```python
from build123d import *

# Parameters (mm, degrees)
CYLINDER011_R     = 1.375
CYLINDER011_DEPTH = 1.4
CYLINDER012_R     = 1.375
CYLINDER012_DEPTH = 1.4
CYLINDER013_R     = 1.375
CYLINDER013_DEPTH = 1.4
CYLINDER010_R     = 1.375
CYLINDER010_DEPTH = 1.4
BOX006_W          = 56
BOX006_H          = 85
BOX006_DEPTH      = 1.4
FILLET002_R       = 3


with BuildPart() as cylinder011:
    # Cylinder011 → Cylinder011 (new body)
    with BuildSketch(Plane(origin=(52.5, 81.5, 9), x_dir=(1, 0, 0), z_dir=(0, 0, 1))):
        Circle(CYLINDER011_R)
    extrude(amount=CYLINDER011_DEPTH)


with BuildPart() as cylinder012:
    # Cylinder012 → Cylinder012 (new body)
    with BuildSketch(Plane(origin=(52.5, 23.5, 9), x_dir=(1, 0, 0), z_dir=(0, 0, 1))):
        Circle(CYLINDER012_R)
    extrude(amount=CYLINDER012_DEPTH)


with BuildPart() as cylinder013:
    # Cylinder013 → Cylinder013 (new body)
    with BuildSketch(Plane(origin=(3.5, 23.5, 9), x_dir=(1, 0, 0), z_dir=(0, 0, 1))):
        Circle(CYLINDER013_R)
    extrude(amount=CYLINDER013_DEPTH)


with BuildPart() as pi_board_holes:
    # Cylinder010 → Cylinder010 (new body)
    with BuildSketch(Plane(origin=(3.5, 81.5, 9), x_dir=(1, 0, 0), z_dir=(0, 0, 1))):
        Circle(CYLINDER010_R)
    extrude(amount=CYLINDER010_DEPTH)

    # Fusion003: union Cylinder011, Cylinder012, Cylinder013
    add(cylinder011.part)
    add(cylinder012.part)
    add(cylinder013.part)


with BuildPart() as pi_base_board:
    # Box006 → Box006 (new body)
    with BuildSketch(Plane.XY.offset(9)):
        with Locations((28, 42.5)):
            Rectangle(BOX006_W, BOX006_H)
    extrude(amount=BOX006_DEPTH)

    # Fillet002
    fillet002_edges = [pi_base_board.edges().sort_by_distance(p)[0] for p in [
        (0, 0, 9.7),
        (0, 85, 9.7),
        (56, 0, 9.7),
        (56, 85, 9.7),
    ]]
    fillet(fillet002_edges, radius=FILLET002_R)

    # Cut002: cut Pi Board Holes
    add(pi_board_holes.part, mode=Mode.SUBTRACT)


with BuildPart() as pi_base_board_1:
    # Cut002 placement: moved
    add(pi_base_board.part.moved(Location((404.8, 35, 0))))


solid = pi_base_board_1.part
```
Geometry: final body of the model. Coordinates: model frame, mm. Coordinates: 2 decimals unless noted, no trailing zeros. Loops run counter-clockwise (first coordinate to the right, second up) from the corner with the lowest first, then second, coordinate; pieces in that order, holes last. Notation, with made-up numbers: M 7.25,-25.75 L 18.25,-25.75 A16 ccw 18.25,4.25 Z; hole C 72,85 d1. An arc over 180 degrees is marked long. Put each result on its own line as item: value.
(1) Material intervals for probe 1 along X at (y, z) = (116.5, 9.4) (3 decimals); probe 2 along Y at (x, z) = (408.3, 9.4) (3 decimals), sorted ascending.
Answer sheet:
probe 1: x = 404.8 to 406.925, 409.675 to 455.925, 458.675 to 460.8
probe 2: y = 35 to 57.125, 59.875 to 115.125, 117.875 to 120
(2) Cut plane A-A on y = 58.5. Return the cut outline in (x, z) (3 decimals), then the cut area to 3 significant figures.
Answer sheet:
outline: M 404.8,9 L 406.925,9 L 406.925,10.4 L 404.8,10.4 Z; M 409.675,9 L 455.925,9 L 455.925,10.4 L 409.675,10.4 Z; M 458.675,9 L 460.8,9 L 460.8,10.4 L 458.675,10.4 Z
area: 70.7 mm^2
(3) Draft query along Y for faces 1 (the face through (405.66, 119.1, 9.71)), 2 (the face through (432, 78, 9)), 3 (the face through (409.612, 58.913, 9.69)). Return one class per face: pulls with the +Y half, pulls with the -Y half, needs draft (parallel to the pull), parting line crosses it, or undercut.
Answer sheet:
face 1: pulls with the +Y half
face 2: needs draft
face 3: undercut
